Input: part model. Units: mm. Frame: model coordinates. A direction names the side the tool comes from. Give positions to 0.01 mm unless a question says otherwise; leave off trailing zeros. Loops run counter-clockwise (first coordinate to the right, second up) from the corner with the lowest first, then second, coordinate; pieces in that order, holes last. Notation, with made-up numbers: M 46.5,-30 L 79.5,-30 A5 ccw 79.5,-23 Z; hole C 58.5,-23 d10. An arc over 180 degrees is marked long. Answer as a JSON object with one key per item and string values. Group by question number.
```python
from build123d import *

# Parameters (mm, degrees)
EXTRUDE_1_DEPTH             = 90
SKETCH_2_W                  = 90
SKETCH_2_H                  = 44.25
EXTRUDE_2_DEPTH             = 8.2
SKETCH_3_W                  = 90
SKETCH_3_H                  = 102.45
EXTRUDE_3_DEPTH             = 8.2
SKETCH_4_W                  = 4.5
SKETCH_4_H                  = 3.95
CUT_EXTRUDE_1_DEPTH         = 91
SKETCH_5_W                  = 2.25
SKETCH_5_H                  = 3.95
CUT_EXTRUDE_2_DEPTH         = 91
SKETCH_6_W                  = 3.95
SKETCH_6_H                  = 2.25
CUT_EXTRUDE_3_DEPTH         = 91
SKETCH_7_W                  = 3.95
SKETCH_7_H                  = 29.5
CUT_EXTRUDE_4_DEPTH         = 91
SKETCH_8_W                  = 3.95
SKETCH_8_H                  = 9
CUT_EXTRUDE_5_DEPTH         = 91
SKETCH_9_W                  = 3.95
SKETCH_9_H                  = 29.5
CUT_EXTRUDE_6_DEPTH         = 91
SKETCH_10_W                 = 3.95
SKETCH_10_H                 = 6.2
CUT_EXTRUDE_7_DEPTH         = 91
SKETCH_11_W                 = 2.25
SKETCH_11_H                 = 3.95
CUT_EXTRUDE_8_DEPTH         = 91
SKETCH_12_W                 = 4.5
SKETCH_12_H                 = 3.95
CUT_EXTRUDE_9_DEPTH         = 91
SKETCH_13_W                 = 9
SKETCH_13_H                 = 3.95
CUT_EXTRUDE_10_DEPTH        = 91
SKETCH_14_W                 = 46.1
SKETCH_14_H                 = 96.1
CUT_EXTRUDE_11_DEPTH        = 86.6
HOLE_WIZARD_2_5_2_5_1_D     = 2.5
HOLE_WIZARD_2_5_2_5_1_DEPTH = 90
HOLE_WIZARD_4_5_4_5_1_D     = 4.5
HOLE_WIZARD_4_5_4_5_1_DEPTH = 90
SKETCH_22_R                 = 1.631577579
SKETCH_22_R_2               = 1.519375383
SKETCH_22_R_3               = 1.487580747
SKETCH_22_R_4               = 1.581735942
SKETCH_22_R_5               = 1.487835557
SKETCH_22_R_6               = 1.42600834
SKETCH_22_R_7               = 1.628129915
SKETCH_22_R_8               = 1.52367125
EXTRUDE_4_DEPTH             = 90
FILLET_5_R                  = 2
FILLET_6_R                  = 2
FILLET_7_R                  = 2
FILLET_8_R                  = 2
FILLET_9_R                  = 2
FILLET_10_R                 = 2
FILLET_11_R                 = 2
FILLET_12_R                 = 2
FILLET_13_R                 = 2
FILLET_14_R                 = 2
FILLET_15_R                 = 2
FILLET_16_R                 = 2
FILLET_17_R                 = 2
FILLET_18_R                 = 2
FILLET_19_R                 = 2
FILLET_20_R                 = 2


with BuildPart() as part:
    # Эскиз1 → Бобышка-Вытянуть1 (new body)
    with BuildSketch(Plane(origin=(90, 0, 0), x_dir=(0, 0, -1), z_dir=(1, 0, 0))):
        with BuildLine():
            Line((6.75, 225.906238208), (6.75, 320.75))
            Line((6.75, 320.75), (-38.093761792, 320.75))
            ThreePointArc((-38.093761792, 320.75), (-41.825, 319.5), (-38.093761792, 318.25))
            Line((-38.093761792, 318.25), (-37.5, 318.25))
            Line((-37.5, 318.25), (-37.5, 284.75))
            Line((-37.5, 284.75), (-38.093761792, 284.75))
            ThreePointArc((-38.093761792, 284.75), (-41.825, 283.5), (-38.093761792, 282.25))
            Line((-38.093761792, 282.25), (-37.5, 282.25))
            Line((-37.5, 282.25), (-37.5, 269.25))
            Line((-37.5, 269.25), (-38.093761792, 269.25))
            ThreePointArc((-38.093761792, 269.25), (-41.825, 268), (-38.093761792, 266.75))
            Line((-38.093761792, 266.75), (-37.5, 266.75))
            Line((-37.5, 266.75), (-37.5, 233.25))
            Line((-37.5, 233.25), (-38.093761792, 233.25))
            ThreePointArc((-38.093761792, 233.25), (-41.825, 232), (-38.093761792, 230.75))
            Line((-38.093761792, 230.75), (-37.5, 230.75))
            Line((-37.5, 230.75), (-37.5, 226.5))
            Line((-37.5, 226.5), (-33.25, 226.5))
            Line((-33.25, 226.5), (-33.25, 225.906238208))
            ThreePointArc((-33.25, 225.906238208), (-32, 222.175), (-30.75, 225.906238208))
            Line((-30.75, 225.906238208), (-30.75, 226.5))
            Line((-30.75, 226.5), (-22.25, 226.5))
            Line((-22.25, 226.5), (-22.25, 225.906238208))
            ThreePointArc((-22.25, 225.906238208), (-21, 222.175), (-19.75, 225.906238208))
            Line((-19.75, 225.906238208), (-19.75, 226.5))
            Line((-19.75, 226.5), (-6.75, 226.5))
            Line((-6.75, 226.5), (-6.75, 225.906238208))
            ThreePointArc((-6.75, 225.906238208), (-5.5, 222.175), (-4.25, 225.906238208))
            Line((-4.25, 225.906238208), (-4.25, 226.5))
            Line((-4.25, 226.5), (4.25, 226.5))
            Line((4.25, 226.5), (4.25, 225.906238208))
            ThreePointArc((4.25, 225.906238208), (5.5, 222.175), (6.75, 225.906238208))
        make_face()
    extrude(amount=-EXTRUDE_1_DEPTH)

    # Эскиз2 → Бобышка-Вытянуть2 (add)
    with BuildSketch(Plane(origin=(0, 320.75, 0), x_dir=(-1, 0, 0), z_dir=(0, 1, 0))):
        with Locations((-45, 15.375)):
            Rectangle(SKETCH_2_W, SKETCH_2_H)
    extrude(amount=EXTRUDE_2_DEPTH)

    # Эскиз3 → Бобышка-Вытянуть3 (add)
    with BuildSketch(Plane(origin=(0, 0, -6.75), x_dir=(-1, 0, 0), z_dir=(0, 0, -1))):
        with Locations((-45, 277.725)):
            Rectangle(SKETCH_3_W, SKETCH_3_H)
    extrude(amount=EXTRUDE_3_DEPTH)

    # Эскиз4 → Вырез-Вытянуть1 (cut, through all)
    with BuildSketch(Plane.ZY):
        with Locations((26.5, 326.975)):
            Rectangle(SKETCH_4_W, SKETCH_4_H)
    extrude(amount=-CUT_EXTRUDE_1_DEPTH, mode=Mode.SUBTRACT)

    # Эскиз5 → Вырез-Вытянуть2 (cut, through all)
    with BuildSketch(Plane.ZY):
        with Locations((36.375, 326.975)):
            Rectangle(SKETCH_5_W, SKETCH_5_H)
    extrude(amount=-CUT_EXTRUDE_2_DEPTH, mode=Mode.SUBTRACT)

    # Эскиз6 → Вырез-Вытянуть3 (cut, through all)
    with BuildSketch(Plane.ZY):
        with Locations((-12.975, 227.625)):
            Rectangle(SKETCH_6_W, SKETCH_6_H)
    extrude(amount=-CUT_EXTRUDE_3_DEPTH, mode=Mode.SUBTRACT)

    # Эскиз7 → Вырез-Вытянуть4 (cut, through all)
    with BuildSketch(Plane.ZY):
        with Locations((-12.975, 250)):
            Rectangle(SKETCH_7_W, SKETCH_7_H)
    extrude(amount=-CUT_EXTRUDE_4_DEPTH, mode=Mode.SUBTRACT)

    # Эскиз8 → Вырез-Вытянуть5 (cut, through all)
    with BuildSketch(Plane.ZY):
        with Locations((-12.975, 275.75)):
            Rectangle(SKETCH_8_W, SKETCH_8_H)
    extrude(amount=-CUT_EXTRUDE_5_DEPTH, mode=Mode.SUBTRACT)

    # Эскиз9 → Вырез-Вытянуть6 (cut, through all)
    with BuildSketch(Plane.ZY):
        with Locations((-12.975, 301.5)):
            Rectangle(SKETCH_9_W, SKETCH_9_H)
    extrude(amount=-CUT_EXTRUDE_6_DEPTH, mode=Mode.SUBTRACT)

    # Эскиз10 → Вырез-Вытянуть7 (cut, through all)
    with BuildSketch(Plane.ZY):
        with Locations((-12.975, 325.85)):
            Rectangle(SKETCH_10_W, SKETCH_10_H)
    extrude(amount=-CUT_EXTRUDE_7_DEPTH, mode=Mode.SUBTRACT)

    # Эскиз11 → Вырез-Вытянуть8 (cut, through all)
    with BuildSketch(Plane.ZY):
        with Locations((-9.875, 326.975)):
            Rectangle(SKETCH_11_W, SKETCH_11_H)
    extrude(amount=-CUT_EXTRUDE_8_DEPTH, mode=Mode.SUBTRACT)

    # Эскиз12 → Вырез-Вытянуть9 (cut, through all)
    with BuildSketch(Plane.ZY):
        with Locations((0, 326.975)):
            Rectangle(SKETCH_12_W, SKETCH_12_H)
    extrude(amount=-CUT_EXTRUDE_9_DEPTH, mode=Mode.SUBTRACT)

    # Эскиз13 → Вырез-Вытянуть10 (cut, through all)
    with BuildSketch(Plane.ZY):
        with Locations((13.25, 326.975)):
            Rectangle(SKETCH_13_W, SKETCH_13_H)
    extrude(amount=-CUT_EXTRUDE_10_DEPTH, mode=Mode.SUBTRACT)

    # Эскиз14 → Вырез-Вытянуть11 (cut)
    with BuildSketch(Plane(origin=(90, 0, 0), x_dir=(0, 0, -1), z_dir=(1, 0, 0))):
        with Locations((-13.25, 275.75)):
            Rectangle(SKETCH_14_W, SKETCH_14_H)
    extrude(amount=-CUT_EXTRUDE_11_DEPTH, mode=Mode.SUBTRACT)

    # Диаметр отверстия Ø2.5 (2.5)1
    with Locations(Plane(origin=(90, 0, 0), x_dir=(0, 0, -1), z_dir=(1, 0, 0))):
        with Locations((-39.75, 232), (-21, 224.25), (-39.75, 283.5), (-5.5, 224.25), (5.5, 224.25), (-39.75, 319.5), (-39.75, 268), (-32, 224.25)):
            Hole(HOLE_WIZARD_2_5_2_5_1_D / 2, depth=HOLE_WIZARD_2_5_2_5_1_DEPTH)

    # Диаметр отверстия Ø4.5 (4.5)1
    with Locations(Plane.ZY):
        with Locations((21, 327.25), (32, 327.25), (-13.25, 232), (-13.25, 268), (-13.25, 283.5), (-13.25, 319.5), (-5.5, 327.25), (5.5, 327.25)):
            Hole(HOLE_WIZARD_4_5_4_5_1_D / 2, depth=HOLE_WIZARD_4_5_4_5_1_DEPTH)

    # Эскиз22 → Бобышка-Вытянуть4 (add)
    with BuildSketch(Plane(origin=(90, 0, 0), x_dir=(0, 0, -1), z_dir=(1, 0, 0))):
        with Locations((-39.75, 319.5)):
            Circle(SKETCH_22_R)
        with Locations((-39.75, 283.5)):
            Circle(SKETCH_22_R_2)
        with Locations((-39.75, 268)):
            Circle(SKETCH_22_R_3)
        with Locations((-39.75, 232)):
            Circle(SKETCH_22_R_4)
        with Locations((-32, 224.25)):
            Circle(SKETCH_22_R_5)
        with Locations((-21, 224.25)):
            Circle(SKETCH_22_R_6)
        with Locations((-5.5, 224.25)):
            Circle(SKETCH_22_R_7)
        with Locations((5.5, 224.25)):
            Circle(SKETCH_22_R_8)
    extrude(amount=-EXTRUDE_4_DEPTH)

    # Скругление5
    fillet_5_edges = [part.edges().sort_by_distance(p)[0] for p in [
        (45, 325, 35.25),
    ]]
    fillet(fillet_5_edges, radius=FILLET_5_R)

    # Скругление6
    fillet_6_edges = [part.edges().sort_by_distance(p)[0] for p in [
        (45, 325, 28.75),
    ]]
    fillet(fillet_6_edges, radius=FILLET_6_R)

    # Скругление7
    fillet_7_edges = [part.edges().sort_by_distance(p)[0] for p in [
        (45, 325, 24.25),
    ]]
    fillet(fillet_7_edges, radius=FILLET_7_R)

    # Скругление8
    fillet_8_edges = [part.edges().sort_by_distance(p)[0] for p in [
        (45, 325, 17.75),
    ]]
    fillet(fillet_8_edges, radius=FILLET_8_R)

    # Скругление9
    fillet_9_edges = [part.edges().sort_by_distance(p)[0] for p in [
        (45, 325, 8.75),
    ]]
    fillet(fillet_9_edges, radius=FILLET_9_R)

    # Скругление10
    fillet_10_edges = [part.edges().sort_by_distance(p)[0] for p in [
        (45, 325, 2.25),
    ]]
    fillet(fillet_10_edges, radius=FILLET_10_R)

    # Скругление11
    fillet_11_edges = [part.edges().sort_by_distance(p)[0] for p in [
        (45, 325, -2.25),
    ]]
    fillet(fillet_11_edges, radius=FILLET_11_R)

    # Скругление12
    fillet_12_edges = [part.edges().sort_by_distance(p)[0] for p in [
        (45, 325, -8.75),
    ]]
    fillet(fillet_12_edges, radius=FILLET_12_R)

    # Скругление13
    fillet_13_edges = [part.edges().sort_by_distance(p)[0] for p in [
        (45, 322.75, -11),
    ]]
    fillet(fillet_13_edges, radius=FILLET_13_R)

    # Скругление14
    fillet_14_edges = [part.edges().sort_by_distance(p)[0] for p in [
        (45, 316.25, -11),
    ]]
    fillet(fillet_14_edges, radius=FILLET_14_R)

    # Скругление15
    fillet_15_edges = [part.edges().sort_by_distance(p)[0] for p in [
        (45, 286.75, -11),
    ]]
    fillet(fillet_15_edges, radius=FILLET_15_R)

    # Скругление16
    fillet_16_edges = [part.edges().sort_by_distance(p)[0] for p in [
        (45, 280.25, -11),
    ]]
    fillet(fillet_16_edges, radius=FILLET_16_R)

    # Скругление17
    fillet_17_edges = [part.edges().sort_by_distance(p)[0] for p in [
        (45, 271.25, -11),
    ]]
    fillet(fillet_17_edges, radius=FILLET_17_R)

    # Скругление18
    fillet_18_edges = [part.edges().sort_by_distance(p)[0] for p in [
        (45, 264.75, -11),
    ]]
    fillet(fillet_18_edges, radius=FILLET_18_R)

    # Скругление19
    fillet_19_edges = [part.edges().sort_by_distance(p)[0] for p in [
        (45, 235.25, -11),
    ]]
    fillet(fillet_19_edges, radius=FILLET_19_R)

    # Скругление20
    fillet_20_edges = [part.edges().sort_by_distance(p)[0] for p in [
        (45, 228.75, -11),
    ]]
    fillet(fillet_20_edges, radius=FILLET_20_R)


solid = part.part
```
1. Section D-D (y = 298). Output: boundary loops of the cut face in (x, z), then the cut area to 3 significant figures.
2. Reachability of faces 1 (the flat face through (46, 323, 37.5)), 2 (the flat face through (47, 323.8, 14)), 3 (the flat face through (44, 301, -11)), 4 (the cylindrical face through (46, 268, -11)) from +Z, -Z, +X, -X, +Y, -Y: full face, straight path, thin tool, end or side. Return the list, or none.
3. First-contact query: P1, Ø1, axis at x = 38.5, z = -14.5, coming from the +Y side; P2, Ø2, axis at x = 32, y = 302, coming from the +Z side; P3, Ø2.5, axis at x = 39, z = 12, coming from the +Y side. Flat tips, straight axial feed; report the tip coordinate or a pass-through.
4. Material intervals for L1, parallel to Z at x = 39, y = 304.5; L2, parallel to Z at x = 38.5, y = 283.5 (3 decimals); L3, parallel to Y at x = 54, z = -0.5, sorted ascending.
5. Section C-C (z = 5.5). Output: boundary loops of the cut face in (x, y) (3 decimals), then the cut area to 3 significant figures.
6. Mould query, pull axis Y, two halves, no side actions, for faces 5 (the flat face through (46, 229, 37.5)), 6 (the cylindrical face through (45.63, 325, -5.42)). Classes: pulls with the +Y half, pulls with the -Y half, needs draft (parallel to the pull), parting line crosses it, or undercut.
7. Section A-A (z = 39.75). Output: boundary loops of the cut face in (x, y) (3 decimals), then the cut area to 3 significant figures.
8. Section B-B (y = 224.25). Output: boundary loops of the cut face in (x, z) (3 decimals).
Geometry results:
{
 "1": {"outline": "M 0,-11 L 90,-11 L 90,-9.8 L 3.4,-9.8 L 3.4,36.3 L 90,36.3 L 90,37.5 L 0,37.5 Z", "area": "373 mm2"},
 "2": {"face 1": "+X, -X, +Y", "face 2": "+X", "face 3": "-Z, +X, -X", "face 4": "+X, -X"},
 "3": {"P1": "y = 322.75", "P2": "z = 37.5", "P3": "y = 325"},
 "4": {"L1": "-11 to -9.8, 36.3 to 37.5", "L2": "-11 to -9.8, 36.3 to 41.825", "L3": "226.5 to 227.7, 323.8 to 325.02"},
 "5": {"outline": "M 0,222.175 L 90,222.175 L 90,227.7 L 3.4,227.7 L 3.4,323.8 L 90,323.8 L 90,325 L 0,325 Z", "area": "932 mm2"},
 "6": {"face 5": "needs draft", "face 6": "undercut"},
 "7": {"outline": "M 0,229.925 L 90,229.925 L 90,234.075 L 0,234.075 Z; M 0,265.925 L 90,265.925 L 90,270.075 L 0,270.075 Z; M 0,281.425 L 90,281.425 L 90,285.575 L 0,285.575 Z; M 0,317.425 L 90,317.425 L 90,321.575 L 0,321.575 Z", "area": "1,490 mm2"},
 "8": {"outline": "M 0,-7.575 L 90,-7.575 L 90,-3.425 L 0,-3.425 Z; M 0,3.425 L 90,3.425 L 90,7.575 L 0,7.575 Z; M 0,18.925 L 90,18.925 L 90,23.075 L 0,23.075 Z; M 0,29.925 L 90,29.925 L 90,34.075 L 0,34.075 Z"}
}
